The figure shows three views and two pictorial views of one solid part (mm, origin at its lowest corner). Answer the questions. Round coordinates to 2 decimals unless told otherwise and drop trailing zeros. Order: outer loops, then holes, each group sorted by start corner. A loop starts at its lowest first (then second) coordinate and runs counter-clockwise, first axis right, second up. Notation, with made-up numbers: M 17,63.5 L 38,63.5 A28 cw 38,98.5 Z; hole C 0,68 d8. An arc over 180 degrees is marked long. Answer as CSV lines item,"result".
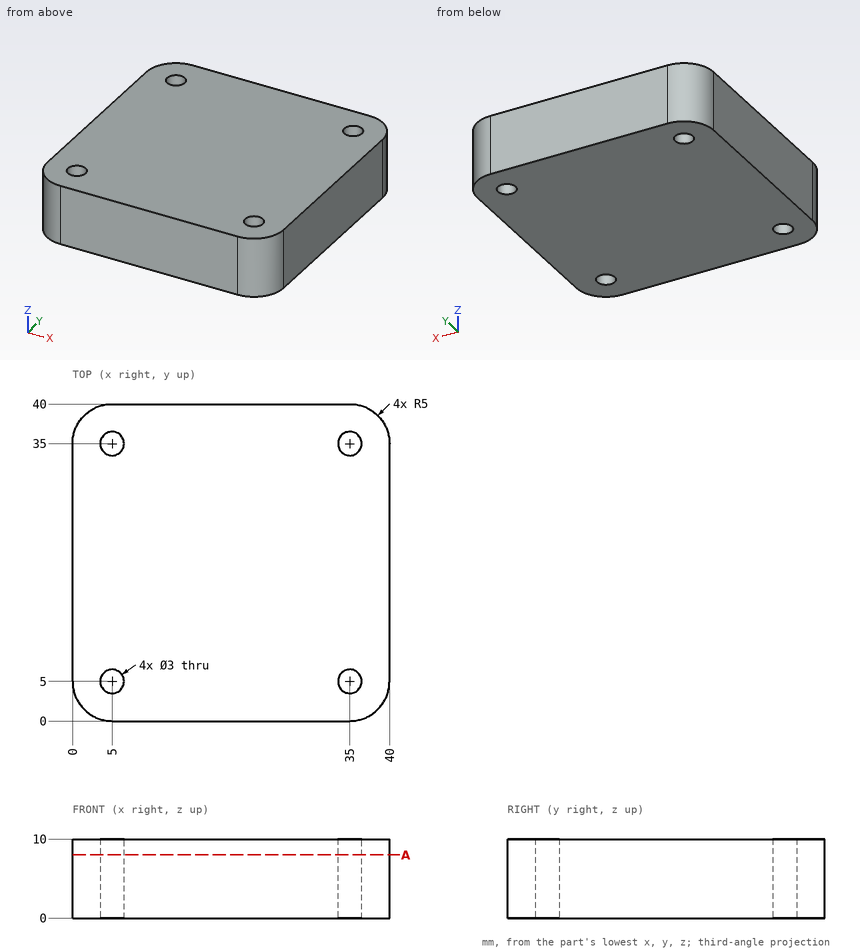
Item 1: Find the intervals of material crossed by probe 1 along Y at (x, z) = (5, 7.75); probe 2 along Y at (x, z) = (6, 1.5); probe 3 along Y at (x, z) = (2, 8.75), in increasing order. Write a range as [from, to].
Ans:
probe 1,"[0, 3.5], [6.5, 33.5], [36.5, 40]"
probe 2,"[0, 3.88], [6.12, 33.88], [36.12, 40]"
probe 3,"[1, 39]"
Item 2: A flat-ended cylindrical pin translates along its axis: pin 1 (1.8 mm diameter, centred on x = 5, y = 35, fed in from -Z). Find the tip coordinate at first contact, or state that the pin passes through.
Ans:
pin 1,"through"
Item 3: A cutting plane is placed at A-A, the plane z = 8. Determine the outline of the cut face in (x, y), and give its area (3 significant figures).
Ans:
outline,"M 0,5 A5 ccw 5,0 L 35,0 A5 ccw 40,5 L 40,35 A5 ccw 35,40 L 5,40 A5 ccw 0,35 Z; hole C 5,5 d3; hole C 5,35 d3; hole C 35,5 d3; hole C 35,35 d3"
area,"1,550 mm2"
